Could you check a few things on this model? Use its own coordinates, in mm. Face numbers are marked on the shaded views. A direction names the side the tool comes from. Coordinates: 2 decimals unless noted, no trailing zeros. Order: outer loops, then holes, each group sorted by start corner. A loop starts at its lowest first (then second) coordinate and runs counter-clockwise, first axis right, second up. Notation, with made-up numbers: (43.25, 50.25) -> (70.25, 50.25) arc R21 cw to (70.25, 68.25) -> close; hole circle Ø8 at (-22.75, 68). An arc over 180 degrees is marked (long way). Use a Markdown table: item, result. Add a question column.
1) Which directions (+Z, -Z, +X, -X, +Y, -Y) give clear straight access to the entire face, cutting with the end or side of a thin tool? Please do the marked faces 1 and 2.
2) If I drill on L1, parallel to Z at x = 9, y = 0.4; L2, parallel to X at y = 4, z = -3; L3, parallel to Y at x = 1, z = 18, over which ranges is the centre line in solid material (lowest first)? Write a range as [from, to].
3) If we section it at D-D (z = 0): Write out the boundary of the cut face in (x, y).
4) If we section it at A-A (z = 10): Write out the boundary of the cut face in (x, y).
5) Will these pins go through, and if not, where does the flat tip stop? pin 1 Ø1.6 at (y, z) = (0.5, -10) entering from -X; pin 2 Ø5 at (x, z) = (8, -15.5) entering from +Y; pin 3 Ø7 at (x, z) = (9, 0) entering from -Y; pin 4 Ø4 at (y, z) = (5, -7) entering from +X.
6) If we section it at C-C (z = 17.5): Write out the boundary of the cut face in (x, y), plus the area to 3 significant figures.
7) If we section it at B-B (y = 9.5): Write out the boundary of the cut face in (x, z), plus the area to 3 significant figures.
```python
from build123d import *

# Parameters (mm, degrees)
EXTRUDE_1_DEPTH     = 22.5
SKETCH_2_R          = 4
SKETCH_2_R_2        = 1.5
CUT_EXTRUDE_1_DEPTH = 45.2
CHAMFER_1_SIZE      = 4
FILLET_1_R          = 1.5
FILLET_2_R          = 3
SKETCH_4_R          = 1.5
CUT_EXTRUDE_2_DEPTH = 19


with BuildPart() as part:
    # Эскиз1 → Бобышка-Вытянуть1 (new body, symmetric)
    with BuildSketch(Plane.XY):
        Polygon((0, 0), (0, 16), (1.5, 16), (1.5, 1.5), (18, 1.5), (18, 0), align=None)
    extrude(amount=EXTRUDE_1_DEPTH, both=True)

    # Эскиз2 → Вырез-Вытянуть1 (cut)
    with BuildSketch(Plane(origin=(0, 1.5, 0), x_dir=(1, 0, 0), z_dir=(0, 1, 0))):
        with Locations((9, 0)):
            Circle(SKETCH_2_R)
        with Locations((9, 18.5)):
            Circle(SKETCH_2_R_2)
        with Locations((9, -18.5)):
            Circle(SKETCH_2_R_2)
        with BuildLine():
            Line((7.5, 8.1), (7.5, 12))
            ThreePointArc((7.5, 12), (9, 13.5), (10.5, 12))
            Line((10.5, 12), (10.5, 8.1))
            ThreePointArc((10.5, 8.1), (9, 6.6), (7.5, 8.1))
        make_face()
        with BuildLine():
            Line((10.5, -12), (10.5, -8.1))
            ThreePointArc((10.5, -8.1), (9, -6.6), (7.5, -8.1))
            Line((7.5, -8.1), (7.5, -12))
            ThreePointArc((7.5, -12), (9, -13.5), (10.5, -12))
        make_face()
    extrude(amount=-CUT_EXTRUDE_1_DEPTH, mode=Mode.SUBTRACT)

    # Фаска1
    chamfer_1_edges = [part.edges().sort_by_distance(p)[0] for p in [
        (0.75, 16, 22.5),
        (0.75, 16, -22.5),
        (18, 0.75, 22.5),
        (18, 0.75, -22.5),
    ]]
    chamfer(chamfer_1_edges, length=CHAMFER_1_SIZE)

    # Скругление1
    fillet_1_edges = [part.edges().sort_by_distance(p)[0] for p in [
        (1.5, 1.5, 0),
    ]]
    fillet(fillet_1_edges, radius=FILLET_1_R)

    # Скругление2
    fillet_2_edges = [part.edges().sort_by_distance(p)[0] for p in [
        (0, 0, 0),
    ]]
    fillet(fillet_2_edges, radius=FILLET_2_R)

    # Эскиз4 → Вырез-Вытянуть2 (cut, through all)
    with BuildSketch(Plane.ZY):
        with Locations((-18.5, 9.5)):
            Circle(SKETCH_4_R)
        with Locations((18.5, 9.5)):
            Circle(SKETCH_4_R)
    extrude(amount=-CUT_EXTRUDE_2_DEPTH, mode=Mode.SUBTRACT)


solid = part.part
```
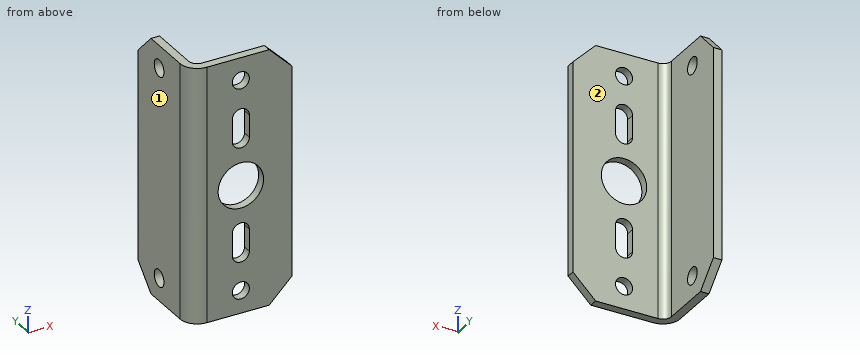
Answer sheet:
| question | item | result |
|---|---|---|
| 1 | face 1 | +Z, -Z, -X, +Y, -Y |
| 1 | face 2 | +Z, -Z, +X, +Y |
| 2 | L1 | [-22.5, -20], [-17, -13.5], [-6.6, -4], [4, 6.6], [13.5, 17], [20, 22.5] |
| 2 | L2 | [0, 1.5] |
| 2 | L3 | [0.76, 8.09], [10.91, 16] |
| 3 | outline | (0, 3) arc R3 ccw to (3, 0) -> (5, 0) -> (5, 1.5) -> (3, 1.5) arc R1.5 cw to (1.5, 3) -> (1.5, 16) -> (0, 16) -> close; (13, 0) -> (18, 0) -> (18, 1.5) -> (13, 1.5) -> close |
| 4 | outline | (0, 3) arc R3 ccw to (3, 0) -> (7.5, 0) -> (7.5, 1.5) -> (3, 1.5) arc R1.5 cw to (1.5, 3) -> (1.5, 16) -> (0, 16) -> close; (10.5, 0) -> (18, 0) -> (18, 1.5) -> (10.5, 1.5) -> close |
| 5 | pin 1 | x = 0.53 |
| 5 | pin 2 | y = 1.5 |
| 5 | pin 3 | through |
| 5 | pin 4 | x = 1.5 |
| 6 | outline | (0, 3) arc R3 ccw to (3, 0) -> (7.88, 0) -> (7.88, 1.5) -> (3, 1.5) arc R1.5 cw to (1.5, 3) -> (1.5, 8.38) -> (0, 8.38) -> close; (0, 10.62) -> (1.5, 10.62) -> (1.5, 16) -> (0, 16) -> close; (10.12, 0) -> (18, 0) -> (18, 1.5) -> (10.12, 1.5) -> close |
| 6 | area | 40.6 mm2 |
| 7 | outline | (0, -22.5) -> (1.5, -22.5) -> (1.5, -20) -> (0, -20) -> close; (0, -17) -> (1.5, -17) -> (1.5, 17) -> (0, 17) -> close; (0, 20) -> (1.5, 20) -> (1.5, 22.5) -> (0, 22.5) -> close |
| 7 | area | 58.5 mm2 |
